```python
from build123d import *

# Parameters (mm, degrees)
F0_R     = 63.5
F1_DEPTH = 79.796453
F3_DEPTH = 40.894
F4_DEPTH = 25.4


with BuildPart() as f1:
    # F0 (on Right) → F1 (new body)
    with BuildSketch(Plane.YZ):
        with Locations((-24.450228, 23.340883)):
            Circle(F0_R)
    extrude(amount=F1_DEPTH)

    # F2 (on face) → F3 (join)
    with BuildSketch(Plane.YZ.offset(79.796453)):
        Polygon((0, 28.579665), (-56.877885, 28.579665), (-56.877885, -11.546232), (0, -11.546232), (0, 8.516717), align=None)
    extrude(amount=-F3_DEPTH)

    # F2 (on face) → F4 (join)
    with BuildSketch(Plane.YZ.offset(79.796453)):
        Polygon((0, 28.579665), (-56.877885, 28.579665), (-56.877885, -11.546232), (0, -11.546232), (0, 8.516717), align=None)
    extrude(amount=F4_DEPTH)


solid = f1.part
```
Geometry: final body of the model. Coordinates: model frame, mm. A direction names the side the tool comes from. Round coordinates to 2 decimals unless told otherwise and drop trailing zeros. Loops run counter-clockwise (first coordinate to the right, second up) from the corner with the lowest first, then second, coordinate; pieces in that order, holes last.
Item 1: Section B-B, the plane z = 5. Output: boundary loops of the cut face in (x, y).
Checked values:
outline: (0, -85.24) - (79.8, -85.24) - (79.8, -56.88) - (105.2, -56.88) - (105.2, 0) - (79.8, 0) - (79.8, 36.34) - (0, 36.34) - close
Item 2: Reachability of faces 1 (the flat face through (92, -56.878, 9)), 2 (the flat face through (92, -28, 28.58)), 3 (the flat face through (92, -29, -11.546)), 4 (the cylindrical face through (39.34, -32.72, 86.3)), 5 (the flat face through (92, 0, 8)) from +Z, -Z, +X, -X, +Y, -Y: full face, straight path, thin tool, end or side. Return the list, or none.
Checked values:
face 1: +Z, -Z, +X, -Y
face 2: +Z, +X, +Y, -Y
face 3: -Z, +X, +Y, -Y
face 4: +X, -X
face 5: +Z, -Z, +X, +Y
Item 3: Contact query for flat-ended pins moving along their axis: P1, Ø1, axis at x = 18.5, z = 48.5, coming from the +Y side; P2, Ø8, axis at x = 74.5, y = 4.5, coming from the -Z side; P3, Ø20.5, axis at x = 93, z = 7, coming from the -Y side. Output: stop coordinate, or through.
Checked values:
P1: stops at y = 34.07
P2: stops at z = -35.05
P3: stops at y = -56.88
Item 4: Section D-D, the plane z = 75. Output: boundary loops of the cut face in (x, y).
Checked values:
outline: (0, -61.38) - (79.8, -61.38) - (79.8, 12.48) - (0, 12.48) - close
Item 5: Section A-A, the plane y = -20. Output: boundary loops of the cut face in (x, z), plus the area to 3 significant figures.
Checked values:
outline: (0, -40) - (79.8, -40) - (79.8, -11.55) - (105.2, -11.55) - (105.2, 28.58) - (79.8, 28.58) - (79.8, 86.68) - (0, 86.68) - close
area: 11,100 mm2
Item 6: Line query: L1, parallel to X at y = -62.5, z = -18.5; L2, parallel to Z at x = 99.5, y = -19; L3, parallel to Z at x = 30, y = 2. Output: solid intervals per line, ascending.
Checked values:
L1: x = 0 to 79.8
L2: z = -11.55 to 28.58
L3: z = -34.39 to 81.07
Item 7: Section C-C, the plane x = 93.5. Output: boundary loops of the cut face in (y, z), plus the area to 3 significant figures.
Checked values:
outline: (-56.88, -11.55) - (0, -11.55) - (0, 28.58) - (-56.88, 28.58) - close
area: 2,280 mm2
